Input: part model. Units: mm. Frame: model coordinates. A direction names the side the tool comes from. Give positions to 0.01 mm unless a question says otherwise; leave off trailing zeros. Order: outer loops, then holes, each group sorted by start corner. A loop starts at its lowest first (then second) coordinate and runs counter-clockwise, first axis right, second up.
Autodesk Inventor part; units mm, degrees
ref_plane "YZ Plane" through (0, 0, 0) normal (1, 0, 0) x (0, 1, 0)
ref_plane "XZ Plane" through (0, 0, 0) normal (0, 1, 0) x (-1, 0, 0)
ref_plane "XY Plane" through (0, 0, 0) normal (0, 0, 1) x (1, 0, 0)
sketch "Эскиз1" plane through (0, 0, 0) normal (0, 0, 1) x (1, 0, 0)
  line L0 (-16.5314, 9.6743) -> (0, 14)
  line L1 (0, 14) -> (17, 9)
  line L2 (17, 9) -> (17, 1.7034)
  line L3 (-67.604, 0) -> (31.1007, 0)
  line L4 (-16.5314, -9.6743) -> (0, -14)
  line L5 (0, -14) -> (17, -9)
  line L6 (17, -9) -> (17, 1.7034)
  arc A0 (-16.5314, 9.6743) -> (-16.5314, -9.6743) centre (-14, 0) ccw
  point P0 (0, 0)
  point P1 (-53.5033, 0)
  dimension "d0" = 10
  dimension "d1" = 31
  dimension "d2" = 28
  dimension "d3" = 14
  dimension "d4" = 18
extrude "Выдавливание1" add sketch "Эскиз1" along normal mid plane 28
sketch "Эскиз2" plane through (0, 0, 0) normal (0, 1, 0) x (-1, 0, 0)
  line L0 (0, 7) -> (24, 7)
  line L1 (24, 7) -> (24, -7)
  line L2 (24, -7) -> (0, -7)
  line L3 (0, -7) -> (0, 7)
  line L4 (24, -14) -> (24, 14)
  point P0 (0, 0)
  point P1 (0, 0)
  dimension "d7" = 14
extrude "Выдавливание2" cut sketch "Эскиз2" along normal through all both and the other way through all
sketch "Эскиз3" plane through (0, 0, 14) normal (0, 0, 1) x (1, 0, 0)
  arc A0 (-16.5314, 9.6743) -> (-16.5314, -9.6743) centre (-14, 0) ccw
  point P0 (0, 0)
hole "Отверстие1" at (-14, 0, 14) direction (0, 0, -1) diameter 12 end through all
sketch "Эскиз4" plane through (17, -9, 14) normal (1, 0, 0) x (0, 0, -1)
  line L0 (28, 18) -> (0, 18)
  line L1 (28, 18) -> (28, 0)
  point P0 (14, 9)
  point P1 (14, 9)
  dimension "d17" = 9
  dimension "d18" = 14
hole "Отверстие2" at (17, 0, 0) direction (-1, 0, 0) diameter 8.376 end through all
chamfer "Фаска1" distance 1.6 angle 45 1 edges at (17, 0, 4.188)
properties part number "05.01.001" material "Iron, Cast"
1) First-contact query: P1, Ø15.5, axis at y = 6, z = -1.5, coming from the -X side; P2, Ø1.5, axis at y = 7.5, z = 3.5, coming from the -X side; P3, Ø1, axis at x = 1, z = 11, coming from the +Y side. Flat tips, straight axial feed; report the tip coordinate or a pass-through.
2) Cut plane D-D (x = -3). Return the cut outline in (y, z) (3 decimals).
3) Reachability of faces 5 (the face through (-7, 0, -7)), 6 (the face through (-8.4, 11.8, -10.5)) from +Z, -Z, +X, -X, +Y, -Y: full face, straight path, thin tool, end or side. Return the list, or none.
4) Cut plane C-C (z = 0). Return the cut outline in (x, y).
5) Cut plane A-A (z = -8.5). Return the cut outline in (x, y).
6) Line query: probe 1 along Z at (x, y) = (-9.5, 8); probe 2 along X at (y, z) = (0, -10.5); probe 3 along Z at (x, y) = (11.25, 0). Output: solid intervals per line, ascending.
7) Cut plane B-B (x = -8.5). Return the cut outline in (y, z), then the cut area to 3 significant figures.
8) Pull-direction query (Y, two-part tool) for faces 1 (the face through (1, 0, 14)), 2 (the face through (-14, 6, -11)), 3 (the face through (-8.4, -11.8, -10.5)), 4 (the face through (7.592, -2.83, 3.087)); classes: pulls with the +Y half, pulls with the -Y half, needs draft (parallel to the pull), parting line crosses it, or undercut.
Geometry says:
1. P1: stops at x = -23.99
1. P2: stops at x = 0
1. P3: stops at y = 13.85
2. outline: (-13.215, -14) - (13.215, -14) - (13.215, -7) - (-13.215, -7) - close; (-13.215, 7) - (13.215, 7) - (13.215, 14) - (-13.215, 14) - close
3. face 5: -X, +Y, -Y
3. face 6: +Z, -Z, -X, +Y
4. outline: (0, -14) - (17, -9) - (17, -5.79) - (15.4, -4.19) - (0, -4.19) - close; (0, 4.19) - (15.4, 4.19) - (17, 5.79) - (17, 9) - (0, 14) - close
5. outline: (-16.53, -9.67) - (0, -14) - (17, -9) - (17, 9) - (0, 14) - (-16.53, 9.67) arc R10 ccw to start; hole circle Ø12 at (-14, 0)
6. probe 1: z = -14 to -7, 7 to 14
6. probe 2: x = -24 to -20, -8 to 17
6. probe 3: z = -14 to -4.19, 4.19 to 14
7. outline: (-11.78, -14) - (-2.4, -14) - (-2.4, -7) - (-11.78, -7) - close; (-11.78, 7) - (-2.4, 7) - (-2.4, 14) - (-11.78, 14) - close; (2.4, -14) - (11.78, -14) - (11.78, -7) - (2.4, -7) - close; (2.4, 7) - (11.78, 7) - (11.78, 14) - (2.4, 14) - close
7. area: 263 mm2
8. face 1: needs draft
8. face 2: undercut
8. face 3: pulls with the -Y half
8. face 4: undercut
